Geometry check sheet. Reference: drawing and pictorial views, mm from the part's lowest x, y, z. A direction names the side the tool comes from. Coordinates: 2 decimals unless noted, no trailing zeros. Write each loop counter-clockwise with the first axis right and the second up, starting at its lowest first coordinate (ties: lowest second). Pieces come first, ordered by that corner, then holes. Notation, with made-up numbers: (-13, 11) - (0, 11) arc R21 ccw to (0, 35) - close; hole circle Ø5 at (83, -22.75). An arc over 180 degrees is marked (long way). Use one line per item in the form item = value. Start each with the question number.
(1) Gauge pin test, flat ends, axial feed: pin 1 Ø4 at (x, y) = (92.5, 9.5) entering from -Z; pin 2 Ø1.4 at (y, z) = (7, 12) entering from +X; pin 3 Ø3 at (y, z) = (8.5, 12.5) entering from -X; pin 4 Ø1 at (x, z) = (56, 74) entering from -Y. Record the tip position at first contact, or that the pin passes through.
(2) Sectioned sample at B-B (y = 12.25). Record the cut outline in (x, z) (1 decimal), and give its area (3 significant figures).
(3) Sectioned sample at A-A (y = 7.5). Record the cut outline in (x, z) (1 decimal), and give its area (3 significant figures).
(4) Material ranges on line 1 (X direction, y = 8, z = 50) (1 decimal); line 2 (Y direction, x = 23, z = 19); line 3 (Z direction, x = 9.5, y = 6.25), recorded low to high. Write a range as [from, to].
(5) Sectioned sample at C-C (x = 62). Record the cut outline in (y, z).
(6) Sectioned sample at D-D (z = 80.5). Record the cut outline in (x, y) (1 decimal).
(7) Tool access check on the marked faces 1, 2, 3 and 4. Record the directions out of +Z, -Z, +X, -X, +Y, -Y that give a thin tool (end or side, any length) a straight path to the whole face; none if there is none.
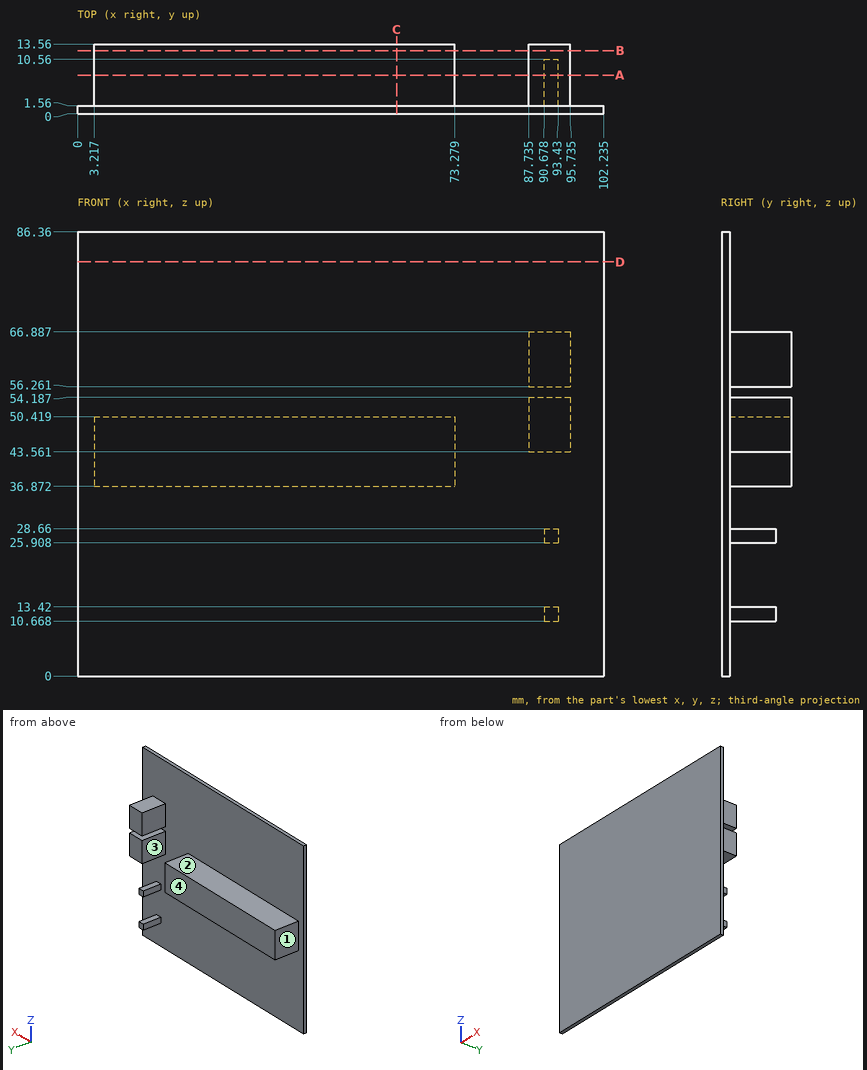
Answers below:
q1.pin_1 = 10.67
q1.pin_2 = 93.43
q1.pin_3 = 90.68
q1.pin_4 = 0
q2.outline = (3.2, 36.9) - (73.3, 36.9) - (73.3, 50.4) - (3.2, 50.4) - close; (87.7, 43.6) - (95.7, 43.6) - (95.7, 54.2) - (87.7, 54.2) - close; (87.7, 56.3) - (95.7, 56.3) - (95.7, 66.9) - (87.7, 66.9) - close
q2.area = 1,120 mm2
q3.outline = (3.2, 36.9) - (73.3, 36.9) - (73.3, 50.4) - (3.2, 50.4) - close; (87.7, 43.6) - (95.7, 43.6) - (95.7, 54.2) - (87.7, 54.2) - close; (87.7, 56.3) - (95.7, 56.3) - (95.7, 66.9) - (87.7, 66.9) - close; (90.7, 10.7) - (93.4, 10.7) - (93.4, 13.4) - (90.7, 13.4) - close; (90.7, 25.9) - (93.4, 25.9) - (93.4, 28.7) - (90.7, 28.7) - close
q3.area = 1,130 mm2
q4.line_1 = [3.2, 73.3], [87.7, 95.7]
q4.line_2 = [0, 1.56]
q4.line_3 = [36.87, 50.42]
q5.outline = (0, 0) - (1.56, 0) - (1.56, 36.87) - (13.56, 36.87) - (13.56, 50.42) - (1.56, 50.42) - (1.56, 86.36) - (0, 86.36) - close
q6.outline = (0, 0) - (102.2, 0) - (102.2, 1.6) - (0, 1.6) - close
q7.face_1 = +Z, -Z, -X, +Y
q7.face_2 = +Z, -X, +Y
q7.face_3 = +Z, -Z, +Y
q7.face_4 = +Z, -Z, +X, -X, +Y
